Could you check a few things on this drawing? It's one solid part, dimensions in mm from its lowest x, y, z. Give positions to 0.01 mm unless a question says otherwise; leave off trailing zeros. Order: outer loops, then holes, each group sorted by start corner. A loop starts at its lowest first (then second) coordinate and runs counter-clockwise, first axis right, second up. Notation, with made-up numbers: (79.25, 42) -> (125.25, 42) arc R24 cw to (125.25, 66) -> close; hole circle Ø1 at (9.5, 88). An arc over 180 degrees is marked (long way). Write each question's results on one line, items separated by ' | '. Start each with the question number.
Q1. Imagine slicing it at A-A, the plane x = 558. Please give me the cut outline in (y, z), then the cut area to 3 significant figures.
Q2. I'm going to push flat-ended pins straight in: pin 1 (2 mm diameter, centred on x = 100, z = 5, fed in from -Y); pin 2 (4 mm diameter, centred on x = 249.5, z = 15.5, fed in from +Y); pin 3 (4 mm diameter, centred on x = 187, z = 3, fed in from -Y). Where does each tip first touch, or does it pass through?
Q3. I need wall thicknesses on line 1 along Y through (x, z) = (473.5, 6.25); line 2 along Y through (x, z) = (145, 6); line 3 along X through (y, z) = (26, 1.25). Which ranges of each line are inside material? Lowest first, please. Write a range as [from, to].
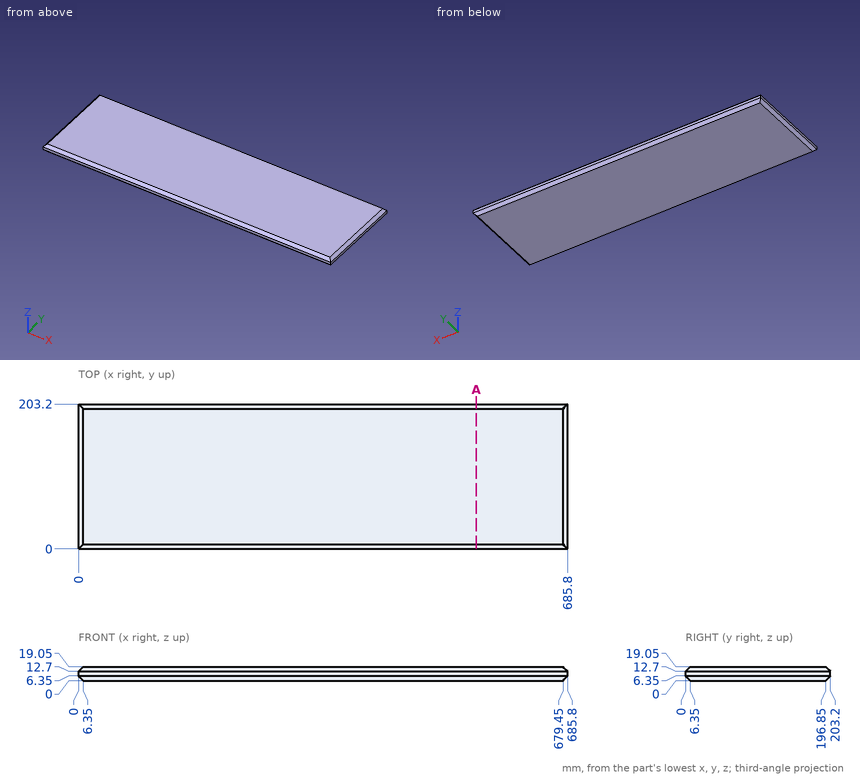
Geometry check:
1) outline: (0, 6.35) -> (6.35, 0) -> (196.85, 0) -> (203.2, 6.35) -> (203.2, 12.7) -> (196.85, 19.05) -> (6.35, 19.05) -> (0, 12.7) -> close | area: 3,790 mm²
2) pin 1: y = 0.35 | pin 2: y = 202.4 | pin 3: y = 1.35
3) line 1: [0.1, 203.1] | line 2: [0.35, 202.85] | line 3: [5.1, 680.7]
